```python
from build123d import *

# Parameters (mm, degrees)
BOSS_EXTRUDE1_DEPTH            = 51
CUT_EXTRUDE1_DEPTH             = 47.5
M3X0_5_TAPPED_HOLE1_D          = 2.5
M3X0_5_TAPPED_HOLE1_DEPTH      = 7.5
M3X0_5_TAPPED_HOLE1_TIP        = 0.751075774
M4_CLEARANCE_HOLE2_D           = 4.5
M4_CLEARANCE_HOLE2_DEPTH       = 4.8
F_13_0_13_DIAMETER_HOLE1_D     = 13
F_13_0_13_DIAMETER_HOLE1_DEPTH = 4.2


with BuildPart() as part:
    # Sketch1 → Boss-Extrude1 (new body)
    with BuildSketch(Plane(origin=(0, 0, 0), x_dir=(1, 0, 0), z_dir=(0, 1, 0))):
        with BuildLine():
            Line((-89.85, 59.75), (89.85, 59.75))
            ThreePointArc((89.85, 59.75), (92.678427125, 58.578427125), (93.85, 55.75))
            Line((93.85, 55.75), (93.85, -55.75))
            ThreePointArc((93.85, -55.75), (92.678427125, -58.578427125), (89.85, -59.75))
            Line((89.85, -59.75), (-89.85, -59.75))
            ThreePointArc((-89.85, -59.75), (-92.678427125, -58.578427125), (-93.85, -55.75))
            Line((-93.85, -55.75), (-93.85, 55.75))
            ThreePointArc((-93.85, 55.75), (-92.678427125, 58.578427125), (-89.85, 59.75))
        make_face()
    extrude(amount=BOSS_EXTRUDE1_DEPTH)

    # Sketch2 → Cut-Extrude1 (cut)
    with BuildSketch(Plane(origin=(0, 51, 0), x_dir=(1, 0, 0), z_dir=(0, 1, 0))):
        with BuildLine():
            Line((-89.05, 51.051250195), (-89.05, -51.051250195))
            ThreePointArc((-89.05, -51.051250195), (-86.117159945, -52.441958359), (-85.181373033, -55.55))
            Line((-85.181373033, -55.55), (-3.968626967, -55.55))
            ThreePointArc((-3.968626967, -55.55), (0, -51.05), (3.968626967, -55.55))
            Line((3.968626967, -55.55), (85.181373033, -55.55))
            ThreePointArc((85.181373033, -55.55), (86.117159945, -52.441958359), (89.05, -51.051250195))
            Line((89.05, -51.051250195), (89.05, 51.051250195))
            ThreePointArc((89.05, 51.051250195), (86.117159945, 52.441958359), (85.181373033, 55.55))
            Line((85.181373033, 55.55), (3.968626967, 55.55))
            ThreePointArc((3.968626967, 55.55), (0, 51.05), (-3.968626967, 55.55))
            Line((-3.968626967, 55.55), (-85.181373033, 55.55))
            ThreePointArc((-85.181373033, 55.55), (-86.117159945, 52.441958359), (-89.05, 51.051250195))
        make_face()
    extrude(amount=-CUT_EXTRUDE1_DEPTH, mode=Mode.SUBTRACT)

    # M3x0.5 Tapped Hole1
    with Locations(Plane(origin=(0, 51, 0), x_dir=(1, 0, 0), z_dir=(0, 1, 0))):
        with Locations((-89.15, 55.05), (-89.15, -55.05), (89.15, -55.05), (89.15, 55.05), (0, -55.05), (0, 55.05)):
            Hole(M3X0_5_TAPPED_HOLE1_D / 2, depth=M3X0_5_TAPPED_HOLE1_DEPTH)
            with Locations((0, 0, -(M3X0_5_TAPPED_HOLE1_DEPTH + M3X0_5_TAPPED_HOLE1_TIP / 2))):  # 118° drill point
                Cone(0, M3X0_5_TAPPED_HOLE1_D / 2, M3X0_5_TAPPED_HOLE1_TIP, mode=Mode.SUBTRACT)

    # M4 Clearance Hole2
    with Locations(Plane.ZY.offset(93.85)):
        with Locations((-39.5, 22), (39.5, 22)):
            Hole(M4_CLEARANCE_HOLE2_D / 2, depth=M4_CLEARANCE_HOLE2_DEPTH)

    # Ø13.0 (13) Diameter Hole1
    with Locations(Plane.XY.offset(59.75)):
        with Locations((43.85, 20)):
            Hole(F_13_0_13_DIAMETER_HOLE1_D / 2, depth=F_13_0_13_DIAMETER_HOLE1_DEPTH)


solid = part.part
```
Read the model definition and answer for the solid it produces. Units are mm, in the model's axes. A direction names the side the tool comes from. Coordinates: 2 decimals unless noted, no trailing zeros. Loops run counter-clockwise (first coordinate to the right, second up) from the corner with the lowest first, then second, coordinate; pieces in that order, holes last. Notation, with made-up numbers: (41.5, 87.5) - (60.5, 87.5) arc R23 ccw to (60.5, 125.5) - close; hole circle Ø7 at (89.25, 50). An arc over 180 degrees is marked (long way). Answer in a Markdown table with one row per item.
1. Determine the mould class of faces 1 (the face through (-1, 25, -59.75)), 2 (the face through (0, 51, -53)), 3 (the face through (44, 28, 55.55)) for opening direction Z: +Z half, -Z half, draft (parallel to the pull), parting line (faces both ways), or undercut.
Conclusion:
| item | result |
|---|---|
| face 1 | -Z half |
| face 2 | draft |
| face 3 | undercut |
2. Straight lines are drawn through the part: line 1 (X direction, y = 46.5, z = -55.05); line 2 (Z direction, x = 89.15, y = 49.5); line 3 (Z direction, x = 89, y = 48). For each, find the intervals that lie inside material, in ascending order.
Conclusion:
| item | result |
|---|---|
| line 1 | x = -93.85 to -90.4, -87.9 to -85.15, -4 to -1.25, 1.25 to 4, 85.15 to 87.9, 90.4 to 93.85 |
| line 2 | z = -59.75 to -56.3, -53.8 to 53.8, 56.3 to 59.75 |
| line 3 | z = -59.75 to -56.29, -53.81 to -51.05, 51.05 to 53.81, 56.29 to 59.75 |
3. Which of the six approach directions +Z, -Z, +X, -X, +Y, -Y give full straight-line access (tool end or side, diameter ignored) to faces 4 (the face through (92.647, 25.143, -58.609)), 5 (the face through (-91.416, 19.804, 39.988)), 6 (the face through (89.05, 28, 1)), 7 (the face through (50.344, 20.286, 57.621))?
Conclusion:
| item | result |
|---|---|
| face 4 | -Z, +X, +Y, -Y |
| face 5 | -X |
| face 6 | +Y |
| face 7 | +Z |
4. Given pin 1 (4 mm diameter, centred on x = 89.15, z = 55.05, fed in from +Y); pin 2 (1.5 mm diameter, centred on x = -39.5, z = 30.5, fed in from +Y); pin 3 (3.5 mm diameter, centred on y = 22, z = 39.5, fed in from -X), each flat-ended and moving along its own axis, determine where each tip first touches the part or whether it passes through.
Conclusion:
| item | result |
|---|---|
| pin 1 | stops at y = 51 |
| pin 2 | stops at y = 3.5 |
| pin 3 | stops at x = 89.05 |
5. Find section C-C, the plane y = 47. Write down the section's boundary in (x, z).
Conclusion:
| item | result |
|---|---|
| outline | (-93.85, -55.75) arc R4 ccw to (-89.85, -59.75) - (89.85, -59.75) arc R4 ccw to (93.85, -55.75) - (93.85, 55.75) arc R4 ccw to (89.85, 59.75) - (-89.85, 59.75) arc R4 ccw to (-93.85, 55.75) - close; hole circle Ø2.5 at (-89.15, -55.05); hole circle Ø2.5 at (-89.15, 55.05); hole (-89.05, -51.05) arc R4 cw to (-85.18, -55.55) - (-3.97, -55.55) arc R4 cw (long way) to (3.97, -55.55) - (85.18, -55.55) arc R4 cw to (89.05, -51.05) - (89.05, 51.05) arc R4 cw to (85.18, 55.55) - (3.97, 55.55) arc R4 cw (long way) to (-3.97, 55.55) - (-85.18, 55.55) arc R4 cw to (-89.05, 51.05) - close; hole circle Ø2.5 at (0, -55.05); hole circle Ø2.5 at (0, 55.05); hole circle Ø2.5 at (89.15, -55.05); hole circle Ø2.5 at (89.15, 55.05) |
6. Find section A-A, the plane x = 43.85. Write down the section's boundary in (y, z), then the cut area to 3 significant figures.
Conclusion:
| item | result |
|---|---|
| outline | (0, -59.75) - (51, -59.75) - (51, -55.55) - (3.5, -55.55) - (3.5, 55.55) - (13.5, 55.55) - (13.5, 59.75) - (0, 59.75) - close; (26.5, 55.55) - (51, 55.55) - (51, 59.75) - (26.5, 59.75) - close |
| area | 763 mm² |
7. Find section B-B, the plane z = 39.5. Write down the section's boundary in (x, y).
Conclusion:
| item | result |
|---|---|
| outline | (-93.85, 0) - (93.85, 0) - (93.85, 51) - (89.05, 51) - (89.05, 3.5) - (-89.05, 3.5) - (-89.05, 19.75) - (-93.85, 19.75) - close; (-93.85, 24.25) - (-89.05, 24.25) - (-89.05, 51) - (-93.85, 51) - close |
8. Find section D-D, the plane y = 22. Count the separate pieces of the cut face and the enclosed holes in it, then the cut area to 3 significant figures.
Conclusion:
| item | result |
|---|---|
| separate pieces | 3 |
| enclosed holes | 0 |
| area | 2,650 mm² |
